Read the model definition and answer for the solid it produces. Units are mm, in the model's axes. Give positions to 0.01 mm unless a question says otherwise; leave off trailing zeros. Order: outer loops, then holes, each group sorted by start corner. A loop starts at its lowest first (then second) coordinate and runs counter-clockwise, first axis right, second up.
```python
from build123d import *

# Parameters (mm, degrees)
SKETCH1_W                                       = 114.3
SKETCH1_H                                       = 101.6
BOSS_EXTRUDE1_DEPTH                             = 3.175
FILLET1_R                                       = 3.175
CSK_FOR_M3_FLAT_HEAD_MACHINE_SCREW1_D           = 3.4
CSK_FOR_M3_FLAT_HEAD_MACHINE_SCREW1_DEPTH       = 7.874
CSK_FOR_M3_FLAT_HEAD_MACHINE_SCREW1_CSINK_D     = 6.3
CSK_FOR_M3_FLAT_HEAD_MACHINE_SCREW1_CSINK_ANGLE = 90
CSK_FOR_M3_FLAT_HEAD_MACHINE_SCREW1_TIP         = 1.021463052
CUT_EXTRUDE1_DEPTH                              = 77.530014537


with BuildPart() as part:
    # Sketch1 → Boss-Extrude1 (new body)
    with BuildSketch(Plane(origin=(0, 0, 0), x_dir=(1, 0, 0), z_dir=(0, 1, 0))):
        Rectangle(SKETCH1_W, SKETCH1_H)
    extrude(amount=BOSS_EXTRUDE1_DEPTH)

    # Fillet1
    fillet1_edges = [part.edges().sort_by_distance(p)[0] for p in [
        (-57.15, 1.5875, -50.8),
        (57.15, 1.5875, -50.8),
        (57.15, 1.5875, 50.8),
        (-57.15, 1.5875, 50.8),
    ]]
    fillet(fillet1_edges, radius=FILLET1_R)

    # CSK for M3 Flat Head Machine Screw1
    with Locations(Plane(origin=(0, 3.175, 0), x_dir=(1, 0, 0), z_dir=(0, 1, 0))):
        with Locations((53.975, -47.625), (53.975, 47.625), (-53.975, 47.625), (-53.975, -47.625)):
            CounterSinkHole(CSK_FOR_M3_FLAT_HEAD_MACHINE_SCREW1_D / 2, CSK_FOR_M3_FLAT_HEAD_MACHINE_SCREW1_CSINK_D / 2, depth=CSK_FOR_M3_FLAT_HEAD_MACHINE_SCREW1_DEPTH, counter_sink_angle=CSK_FOR_M3_FLAT_HEAD_MACHINE_SCREW1_CSINK_ANGLE)
            with Locations((0, 0, -(CSK_FOR_M3_FLAT_HEAD_MACHINE_SCREW1_DEPTH + CSK_FOR_M3_FLAT_HEAD_MACHINE_SCREW1_TIP / 2))):  # 118° drill point
                Cone(0, CSK_FOR_M3_FLAT_HEAD_MACHINE_SCREW1_D / 2, CSK_FOR_M3_FLAT_HEAD_MACHINE_SCREW1_TIP, mode=Mode.SUBTRACT)

    # Sketch4 → Cut-Extrude1 (cut, through all)
    with BuildSketch(Plane(origin=(0, 3.175, 0), x_dir=(1, 0, 0), z_dir=(0, 1, 0))):
        with BuildLine():
            Line((-41.91, -31.75), (-41.91, 31.75))
            ThreePointArc((-41.91, 31.75), (-34.29, 39.37), (-26.67, 31.75))
            Line((-26.67, 31.75), (-26.67, -31.75))
            ThreePointArc((-26.67, -31.75), (-34.29, -39.37), (-41.91, -31.75))
        make_face()
        with BuildLine():
            Line((41.91, -31.75), (41.91, 31.75))
            ThreePointArc((41.91, 31.75), (34.29, 39.37), (26.67, 31.75))
            Line((26.67, 31.75), (26.67, -31.75))
            ThreePointArc((26.67, -31.75), (34.29, -39.37), (41.91, -31.75))
        make_face()
    extrude(amount=-CUT_EXTRUDE1_DEPTH, mode=Mode.SUBTRACT)


solid = part.part
```
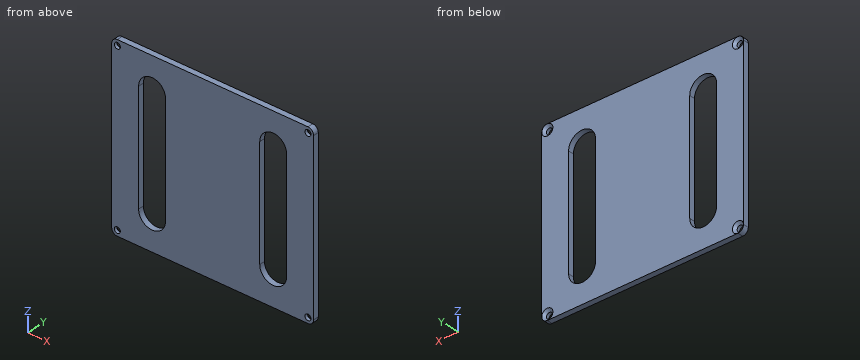
1) Consider L1, parallel to X at y = 2.45, z = -25.5; L2, parallel to X at y = 2.65, z = -37; L3, parallel to Z at x = -28, y = 1.2. Determine where each line is inside the solid, lowest interval first.
Final values:
L1: x = -57.15 to -41.91, -26.67 to 26.67, 41.91 to 57.15
L2: x = -57.15 to -39.81, -28.77 to 28.77, 39.81 to 57.15
L3: z = -50.8 to -36.05, 36.05 to 50.8
2) The part is cut by section B-B on z = 28.5. Determine the outline of the cut face in (x, y) (3 decimals), and give its area (3 significant figures).
Final values:
outline: (-57.15, 0) - (-41.91, 0) - (-41.91, 3.175) - (-57.15, 3.175) - close; (-26.67, 0) - (26.67, 0) - (26.67, 3.175) - (-26.67, 3.175) - close; (41.91, 0) - (57.15, 0) - (57.15, 3.175) - (41.91, 3.175) - close
area: 266 mm2
3) The part is cut by section A-A on x = -34.29. Determine the outline of the cut face in (y, z) (3 decimals), and give its area (3 significant figures).
Final values:
outline: (0, -50.8) - (3.175, -50.8) - (3.175, -39.37) - (0, -39.37) - close; (0, 39.37) - (3.175, 39.37) - (3.175, 50.8) - (0, 50.8) - close
area: 72.6 mm2
